from build123d import *

# Parameters (mm, degrees)
SKETCH3_R            = 12.7
SKETCH3_R_2          = 11.049
BOSS_EXTRUDE1_DEPTH  = 127
SWEEP1_START         = -50.8
SWEEP1_OUTLINE_R     = 12.7
SWEEP1_OUTLINE_R_2   = 11.049
SWEEP1_DEPTH         = 25.4
SWEEP1_2_OUTLINE_R   = 12.7
SWEEP1_2_OUTLINE_R_2 = 11.049
SWEEP1_2_ANGLE       = 90


with BuildPart() as part:
    # Sketch3 → Boss-Extrude1 (new, symmetric)
    with BuildSketch(Plane(origin=(0, 0, 0), x_dir=(0, 0, -1), z_dir=(1, 0, 0))):
        Circle(SKETCH3_R)
        Circle(SKETCH3_R_2, mode=Mode.SUBTRACT)
    extrude(amount=BOSS_EXTRUDE1_DEPTH, both=True)



with BuildPart() as body_2:
    # Sweep1: read off the stored shape, not the designer's step
    # Sweep1 outline → Sweep1 (new body)
    with BuildSketch(Plane(origin=(0, 0, 0), x_dir=(1, 0, 0), z_dir=(0, 1, 0)).offset(SWEEP1_START)):
        with Locations((-152.4, 0)):
            Circle(SWEEP1_OUTLINE_R)
        with Locations((-152.4, 0)):
            Circle(SWEEP1_OUTLINE_R_2, mode=Mode.SUBTRACT)
    extrude(amount=SWEEP1_DEPTH)


with BuildPart() as part_1:
    add(part.part)

    add(body_2.part)  # Sweep1 2 merges body 2
    # Sweep1 2 outline → Sweep1 2 (revolve)
    with BuildSketch(Plane(origin=(-127, -25.4, 0), x_dir=(0, 1, 0), z_dir=(1, 0, 0))):
        with Locations((25.4, 0)):
            Circle(SWEEP1_2_OUTLINE_R)
        with Locations((25.4, 0)):
            Circle(SWEEP1_2_OUTLINE_R_2, mode=Mode.SUBTRACT)
    revolve(axis=Axis((-127, -25.4, 0), (0, 0, 1)), revolution_arc=SWEEP1_2_ANGLE)


solid = part_1.part
Design review of the part built by this model. Coordinates are the model's own, in mm. A direction names the side the tool comes from. Round coordinates to 2 decimals unless told otherwise and drop trailing zeros. Write each loop counter-clockwise with the first axis right and the second up, starting at its lowest first coordinate (ties: lowest second). Pieces come first, ordered by that corner, then holes. Notation, with made-up numbers: M 35.25,8 L 49.25,8 A24 ccw 49.25,41 Z; hole C 62,-1.5 d7. An arc over 180 degrees is marked long. One line per item, written item: value. Start each with the question number.
1. Draft analysis for pull direction Y (two halves, no side actions). For faces 1 (the face through (-1.778, 10.955, 1.438)), 2 (the face through (-165.088, -38.278, -0.558)), 3 (the face through (1.78, -12.4, 2.75)), 4 (the face through (-162, -50.8, -6)), state which applies: pulls with the +Y half, pulls with the -Y half, needs draft (parallel to the pull), parting line crosses it, or undercut.
2. Take a section at B-B on x = 85.5. State the section outline as (y, z) points.
3. Clearance check with flat-ended pins moving along their axes: P1, Ø6, axis at y = -2.5, z = -8, coming from the -X side; P2, Ø4, axis at y = -11, z = 8, coming from the +X side; P3, Ø1, axis at y = -34, z = 3.5, coming from the +X side; P4, Ø6, axis at y = -27, z = 0, coming from the +X side. State where each tip first meets the part, or that it passes through.
4. To check wall thickness, follow probe 1 along Y at (x, z) = (-98, -1); probe 2 along X at (y, z) = (-43, 0); probe 3 along Z at (x, y) = (62, 0). State the ranges of each line that lie inside material, in increasing order. Write a range as from..to.
5. Take a section at A-A on z = 0. State the section outline as (x, y) points, then the cut area to 3 significant figures.
6. Take a section at C-C on y = -37. State the section outline as (x, z) points, then the cut area to 3 significant figures.
7. For faces 5 (the face through (-163.44, -38.28, -0.49)), 6 (the face through (127, -11.2, 1)), list the 3-axis set-ups (+Z, -Z, +X, -X, +Y, -Y) from which the entire face can be reached by the end or side of a thin tool; tool diameter is ignored.
Computed:
1. face 1: undercut
1. face 2: needs draft
1. face 3: parting line crosses it
1. face 4: pulls with the -Y half
2. outline: C 0,0 d25.4; hole C 0,0 d22.1
3. P1: stops at x = -157.2
3. P2: stops at x = 127
3. P3: stops at x = -140.06
3. P4: stops at x = -139.62
4. probe 1: y = -12.66..-11, 11..12.66
4. probe 2: x = -165.1..-163.45, -141.35..-139.7
4. probe 3: z = -12.7..-11.05, 11.05..12.7
5. outline: M -165.1,-50.8 L -163.45,-50.8 L -163.45,-25.4 A36.45 cw -127,11.05 L 127,11.05 L 127,12.7 L -127,12.7 A38.1 ccw -165.1,-25.4 Z; M -141.35,-50.8 L -139.7,-50.8 L -139.7,-25.4 A12.7 cw -127,-12.7 L 127,-12.7 L 127,-11.05 L -127,-11.05 A14.35 ccw -141.35,-25.4 Z
5. area: 1,050 mm²
6. outline: C -152.4,0 d25.4; hole C -152.4,0 d22.1
6. area: 123 mm²
7. face 5: -Y
7. face 6: +Z, -Z, +X, +Y, -Y
